For this review, take the finished solid that the model builds, in its own axes (mm). Face numbers are marked on the shaded views. A direction names the side the tool comes from. Round coordinates to 2 decimals unless told otherwise and drop trailing zeros. Write each loop counter-clockwise with the first axis right and the second up, starting at its lowest first coordinate (ties: lowest second). Pieces come first, ordered by that corner, then holes. Notation, with made-up numbers: (-16, -22) -> (43, -22) arc R11 ccw to (43, -7) -> close; hole circle Ø10 at (-26.5, 8). An arc over 180 degrees is marked (long way). Answer in a Markdown table with one row per item.
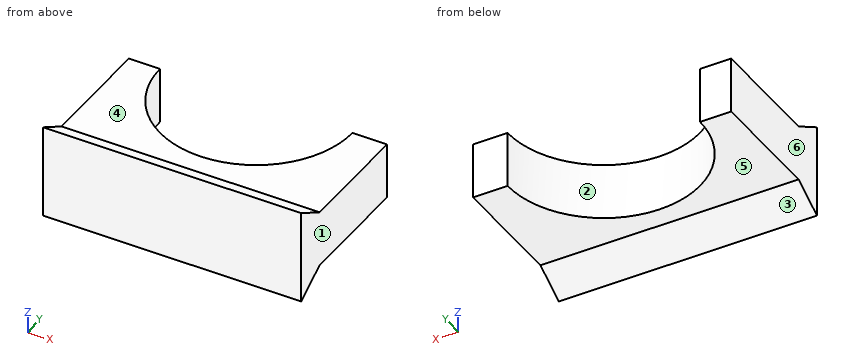
from build123d import *

# Parameters (mm, degrees)
SKETCH1_W           = 139.7
SKETCH1_H           = 76.2
BOSS_EXTRUDE1_DEPTH = 50.8
CUT_EXTRUDE1_DEPTH  = 140.7
SKETCH3_W           = 139.7
SKETCH3_H           = 15.24
BOSS_EXTRUDE2_DEPTH = 63.5
CUT_EXTRUDE4_DEPTH  = 63.5


with BuildPart() as part:
    # Sketch1 → Boss-Extrude1 (new body)
    with BuildSketch(Plane.XY):
        with Locations((69.85, 38.1)):
            Rectangle(SKETCH1_W, SKETCH1_H)
    extrude(amount=BOSS_EXTRUDE1_DEPTH)

    # Sketch2 → Cut-Extrude1 (cut, through all)
    with BuildSketch(Plane(origin=(139.7, 0, 0), x_dir=(0, 0, -1), z_dir=(1, 0, 0))):
        Polygon((-50.8, 76.2), (-50.8, 0), (-40.64, 17.335178993), (-25.4, 17.335178993), (-10.16, 17.335178993), (0, 0), (0, 76.2), align=None)
    extrude(amount=-CUT_EXTRUDE1_DEPTH, mode=Mode.SUBTRACT)

    # Sketch3 → Boss-Extrude2 (add)
    with BuildSketch(Plane(origin=(0, 17.335178993, 0), x_dir=(1, 0, 0), z_dir=(0, 1, 0))):
        with Locations((69.85, -33.02)):
            Rectangle(SKETCH3_W, SKETCH3_H)
        with Locations((69.85, -17.78)):
            Rectangle(SKETCH3_W, SKETCH3_H)
    extrude(amount=BOSS_EXTRUDE2_DEPTH)

    # Sketch7 → Cut-Extrude4 (cut)
    with BuildSketch(Plane.XY.offset(40.64)):
        with BuildLine():
            Line((16.865330571, 80.835178993), (121.005330571, 80.835178993))
            ThreePointArc((121.005330571, 80.835178993), (68.935330571, 28.765178993), (16.865330571, 80.835178993))
        make_face()
    extrude(amount=-CUT_EXTRUDE4_DEPTH, mode=Mode.SUBTRACT)


solid = part.part
1) For line 1 (X direction, y = 47.5, z = 40); line 2 (X direction, y = 41, z = 27); line 3 (Z direction, x = 131, y = 22), list the stretches that pass through material, from the lowest coordinate up. Write a range as [from, to].
Solved:
| item | result |
|---|---|
| line 1 | [0, 28.93], [108.94, 139.7] |
| line 2 | [0, 35.4], [102.47, 139.7] |
| line 3 | [10.16, 40.64] |
2) Consider section B-B on z = 12.5. State the section outline as (x, y) points, then the cut area to 3 significant figures.
Solved:
| item | result |
|---|---|
| outline | (0, 0) -> (139.7, 0) -> (139.7, 80.84) -> (121.01, 80.84) arc R52.07 cw to (16.87, 80.84) -> (0, 80.84) -> close |
| area | 7,030 mm² |
3) Consider section D-D on y = 64.5. State the section outline as (x, z) points.
Solved:
| item | result |
|---|---|
| outline | (0, 10.16) -> (19.49, 10.16) -> (19.49, 40.64) -> (0, 40.64) -> close; (118.38, 10.16) -> (139.7, 10.16) -> (139.7, 40.64) -> (118.38, 40.64) -> close |
4) Mouldability with a two-part tool opening along X and no side actions: class the marked faces 1, 2 and 3 as pulls with the +X half, pulls with the -X half, needs draft (parallel to the pull), parting line crosses it, or undercut.
Solved:
| item | result |
|---|---|
| face 1 | pulls with the +X half |
| face 2 | undercut |
| face 3 | needs draft |
5) Consider section C-C on x = 100.5. State the section outline as (y, z) points, then the cut area to 3 significant figures.
Solved:
| item | result |
|---|---|
| outline | (0, 0) -> (17.34, 10.16) -> (39.42, 10.16) -> (39.42, 40.64) -> (17.34, 40.64) -> (0, 50.8) -> close |
| area | 1,380 mm² |
6) For the marked faces 4, 5 and 6, list the 3-axis set-ups (+Z, -Z, +X, -X, +Y, -Y) from which the entire face can be reached by the end or side of a thin tool; tool diameter is ignored.
Solved:
| item | result |
|---|---|
| face 4 | +Z, +X, -X, +Y |
| face 5 | -Z, +X, -X, +Y |
| face 6 | +Z, -Z, -X, +Y, -Y |
7) Clearance check with flat-ended pins moving along their axes: pin 1 Ø4 at (x, z) = (62.5, 13) entering from +Y; pin 2 Ø8 at (x, y) = (98, 13.5) entering from -Z; pin 3 Ø1.5 at (x, y) = (45.5, 12.5) entering from +Z; pin 4 Ø8 at (x, y) = (79, 36.5) entering from -Z. State where each tip first meets the part, or that it passes through.
Solved:
| item | result |
|---|---|
| pin 1 | y = 29.45 |
| pin 2 | z = 5.57 |
| pin 3 | z = 43.91 |
| pin 4 | through |
8) Consider section A-A on y = 33. State the section outline as (x, z) points, then the cut area to 3 significant figures.
Solved:
| item | result |
|---|---|
| outline | (0, 10.16) -> (48.37, 10.16) -> (48.37, 40.64) -> (0, 40.64) -> close; (89.5, 10.16) -> (139.7, 10.16) -> (139.7, 40.64) -> (89.5, 40.64) -> close |
| area | 3,000 mm² |
